from build123d import *

# Parameters (mm, degrees)
F0_W     = 85.953310132
F0_H     = 118.7221929431
F1_DEPTH = 101.6
F3_T     = -2.54
F4_R     = 0.254
F2_W     = 81.6747397184
F2_H     = 111.1846715212
F5_DEPTH = 76.2


with BuildPart() as f1:
    # F0 (on Front) → F1 (new body)
    with BuildSketch(Plane.XZ):
        with Locations((5.494184792, 0.4023127258)):
            Rectangle(F0_W, F0_H)
    extrude(amount=F1_DEPTH)

    # F3
    f3_openings = [f1.faces().sort_by_distance(p)[0] for p in [
        (5.494185, -101.6, 0.402313),
    ]]
    offset(amount=F3_T, openings=f3_openings)

    # F4
    f4_edges = [f1.edges().sort_by_distance(p)[0] for p in [
        (48.47084, -101.6, 0.402313),
        (5.494185, -101.6, 57.223409),
        (-34.94247, -101.6, 0.402313),
        (5.494185, -101.6, -56.418784),
    ]]
    fillet(f4_edges, radius=F4_R)

    # F2 (on Front) → F5 (join)
    with BuildSketch(Plane.XZ):
        with Locations((-78.1854763627, 0.9429827332)):
            Rectangle(F2_W, F2_H)
    extrude(amount=F5_DEPTH)


solid = f1.part
The listing builds one solid part. Answer for the finished solid, in the listing's coordinates (mm). A direction names the side the tool comes from. Coordinates: 2 decimals unless noted, no trailing zeros. Order: outer loops, then holes, each group sorted by start corner. A loop starts at its lowest first (then second) coordinate and runs counter-clockwise, first axis right, second up. Notation, with made-up numbers: M 24,-8 L 61,-8 A30 ccw 61,24 Z; hole C -4.5,13 d1. An arc over 180 degrees is marked long. Use CSV: the item, a comma, the result in double quotes.
Q1. Given pin 1 Ø24.5 at (x, z) = (-88, -12.5) entering from -Y; pin 2 Ø10 at (x, z) = (-0.5, 12) entering from -Y; pin 3 Ø8 at (x, y) = (-91, -19.5) entering from -Z, each flat-ended and moving along its own axis, determine where each tip first touches the part or whether it passes through.
Here are the results:
pin 1,"y = -76.2"
pin 2,"y = -2.54"
pin 3,"z = -54.65"
Q2. Determine the mould class of faces 4 (the flat face through (5, -51, 57.223)), 5 (the flat face through (-79, -76.2, 2)), 6 (the flat face through (5, -2.54, 1)), 7 (the flat face through (-79, -38, 56.535)) for opening direction Z: pulls with the +Z half, pulls with the -Z half, needs draft (parallel to the pull), parting line crosses it, or undercut.
Here are the results:
face 4,"undercut"
face 5,"needs draft"
face 6,"undercut"
face 7,"pulls with the +Z half"
Q3. Section C-C (x = 21) is taken. Determine the outline of the cut face in (y, z), then the cut area to 3 significant figures.
Here are the results:
outline,"M -101.6,-58.96 L 0,-58.96 L 0,59.76 L -101.6,59.76 L -101.6,57.48 A0.25 ccw -101.35,57.22 L -2.54,57.22 L -2.54,-56.42 L -101.35,-56.42 A0.25 ccw -101.6,-56.67 Z"
area,"805 mm2"
Q4. Section D-D (x = -65.5) is taken. Determine the outline of the cut face in (y, z).
Here are the results:
outline,"M -76.2,-54.65 L 0,-54.65 L 0,56.54 L -76.2,56.54 Z"
Q5. Straight lines are drawn through the part: L1, parallel to Z at x = -15.5, y = -51.5; L2, parallel to X at y = -75, z = 19; L3, parallel to X at y = -89, z = -28.5. For each, find the intervals that lie inside material, in ascending order.
Here are the results:
L1,"-58.96 to -56.42, 57.22 to 59.76"
L2,"-119.02 to -34.94, 45.93 to 48.47"
L3,"-37.48 to -34.94, 45.93 to 48.47"
Q6. Section B-B (z = 2) is taken. Determine the outline of the cut face in (x, y), then the cut area to 3 significant figures.
Here are the results:
outline,"M -119.02,-76.2 L -37.48,-76.2 L -37.48,-101.6 L -35.2,-101.6 A0.25 ccw -34.94,-101.35 L -34.94,-2.54 L 45.93,-2.54 L 45.93,-101.6 L 48.22,-101.6 A0.25 ccw 48.47,-101.35 L 48.47,0 L -119.02,0 Z"
area,"6,930 mm2"
Q7. Section A-A (y = -34.5) is taken. Determine the outline of the cut face in (x, z).
Here are the results:
outline,"M -119.02,-54.65 L -37.48,-54.65 L -37.48,-58.96 L 48.47,-58.96 L 48.47,59.76 L -37.48,59.76 L -37.48,56.54 L -119.02,56.54 Z; hole M -34.94,-56.42 L 45.93,-56.42 L 45.93,57.22 L -34.94,57.22 Z"
Q8. A tool of negligible diameter and unlimited length cuts with its end or side. For faces 1 (the flat face through (5, -101.6, 58)), 2 (the flat face through (45.931, -51, 0)), 3 (the flat face through (-79, -38, -54.649)), from which of +Z, -Z, +X, -X, +Y, -Y can it reach the whole face along a straight path? Write none if from no direction.
Here are the results:
face 1,"+Z, -Z, +X, -X, -Y"
face 2,"-Y"
face 3,"-Z, -X, +Y, -Y"
